from build123d import *

# Parameters (mm, degrees)
SKETCH_2_W                       = 400
SKETCH_2_H                       = 100
SM_BASE_FLANGE_1_DEPTH           = 3
SM_EDGE_FLANGE_1_STRIP_W         = 46
SM_EDGE_FLANGE_1_STRIP_H         = 3
SM_EDGE_FLANGE_1_STRIP_CUT_DEPTH = 400
SM_EDGE_FLANGE_1_DEPTH           = 400


# Sheet-metal steps are written as plain solids
with BuildPart() as part:
    # Sketch 2 → 基体-法兰1 (new body)
    with BuildSketch(Plane.XY):
        Rectangle(SKETCH_2_W, SKETCH_2_H)
    extrude(amount=-SM_BASE_FLANGE_1_DEPTH)

    # 边线-法兰1 strip (across the edge) → 边线-法兰1 strip cut (cut)
    with BuildSketch(Plane(origin=(-200, -50, 0), x_dir=(0, 1, 0), z_dir=(1, 0, 0))):
        with Locations((-3, -1.5)):
            Rectangle(SM_EDGE_FLANGE_1_STRIP_W, SM_EDGE_FLANGE_1_STRIP_H)
    extrude(amount=SM_EDGE_FLANGE_1_STRIP_CUT_DEPTH, mode=Mode.SUBTRACT)

    # 边线-法兰1 section (across the edge) → 边线-法兰1 (add)
    with BuildSketch(Plane(origin=(-200, -50, 0), x_dir=(0, 1, 0), z_dir=(1, 0, 0))):
        with BuildLine():
            Line((0, 17), (0, 97))
            Line((0, 97), (3, 97))
            Line((3, 97), (3, 17))
            ThreePointArc((3, 17), (7.97918472, 4.97918472), (20, 0))
            Line((20, 0), (20, -3))
            ThreePointArc((20, -3), (5.857864376, 2.857864376), (0, 17))
        make_face()
    extrude(amount=SM_EDGE_FLANGE_1_DEPTH)


solid = part.part
Model file for the job. Use its own axes, mm. A direction names the side the tool comes from. Coordinates: 2 decimals unless noted, no trailing zeros. Loops run counter-clockwise (first coordinate to the right, second up) from the corner with the lowest first, then second, coordinate; pieces in that order, holes last. Notation, with made-up numbers: (-12, 50) -> (29, 50) arc R31 ccw to (29, 83) -> close; hole circle Ø1 at (-1, 86). An arc over 180 degrees is marked (long way). Use one line per item in the form item = value. Start each with the question number.
(1) Cut at B-B on y = 40. Give the cut face in (x, z), and give its area (3 significant figures).
(2) Tool access for faces 1 (the flat face through (-3, 11, 0)), 2 (the flat face through (-3, 11, -3)): list every direction of +Z, -Z, +X, -X, +Y, -Y with a clear straight run to the whole face (end or side of a thin tool).
(3) Pull direction X, two halves, no side cores. Call faces 3 (the cylindrical face through (-2.8, -43.986, 2.703)), 4 (the flat face through (-200, -22, -1)), 5 (the flat face through (200, -22, -1)): pulls with the +X half, pulls with the -X half, needs draft (parallel to the pull), parting line crosses it, or undercut.
(4) Probe probe 1 along Z at (x, y) = (-64.5, 31); probe 2 along Y at (x, z) = (110.5, 90.5); probe 3 along Z at (x, y) = (-89, -45). List the from-to ranges inside material, lowest first. Write a range as from..to.
(5) Cut at C-C on z = 37. Give the cut face in (x, y).
(6) Cut at A-A on x = -145. Give the cut face in (y, z).
(7) Flat gauge pins, fed straight in: pin 1 (1.5 mm diameter, centred on x = 148.5, z = 21.5, fed in from +Y); pin 2 (8 mm diameter, centred on x = 55.5, y = 25, fed in from +Z); pin 3 (8 mm diameter, centred on x = 87.5, z = 11, fed in from +Y). Where does each tip first touch, or does it go through?
Values:
q1.outline = (-200, -3) -> (200, -3) -> (200, 0) -> (-200, 0) -> close
q1.area = 1,200 mm2
q2.face_1 = +Z, +X, -X, +Y
q2.face_2 = -Z, +X, -X, +Y, -Y
q3.face_3 = needs draft
q3.face_4 = pulls with the -X half
q3.face_5 = pulls with the +X half
q4.probe_1 = -3..0
q4.probe_2 = -50..-47
q4.probe_3 = 3.77..9
q5.outline = (-200, -50) -> (200, -50) -> (200, -47) -> (-200, -47) -> close
q6.outline = (-50, 17) arc R20 ccw to (-30, -3) -> (50, -3) -> (50, 0) -> (-30, 0) arc R17 cw to (-47, 17) -> (-47, 97) -> (-50, 97) -> close
q7.pin_1 = -47
q7.pin_2 = 0
q7.pin_3 = -43.75
